Build history of the part. All positions in model axes, mm. A direction names the side the tool comes from. Give positions to 0.01 mm unless a question says otherwise; leave off trailing zeros. Write each loop counter-clockwise with the first axis right and the second up, starting at its lowest first coordinate (ties: lowest second). Pieces come first, ordered by that corner, then holes. Notation, with made-up numbers: M 86.5,65.5 L 120.5,65.5 A18 ccw 120.5,71.5 Z; hole C 26,-31.5 d8. An arc over 180 degrees is marked long. One line per item, written item: value. Start each with the question number.
Autodesk Inventor part; units mm, degrees
ref_plane "YZ Plane" through (0, 0, 0) normal (1, 0, 0) x (0, 1, 0)
ref_plane "XZ Plane" through (0, 0, 0) normal (0, 1, 0) x (-1, 0, 0)
ref_plane "XY Plane" through (0, 0, 0) normal (0, 0, 1) x (1, 0, 0)
sketch "Sketch1" plane through (0, 0, 0) normal (0, 0, 1) x (1, 0, 0)
  line L0 (-17.5, -18) -> (17.5, -18)
  line L1 (17.5, -18) -> (17.5, 18)
  line L2 (17.5, 18) -> (-17.5, 18)
  line L3 (-17.5, 18) -> (-17.5, -18)
  line L4 (-17.5, -18) -> (17.5, 18) construction
  line L5 (17.5, -18) -> (-17.5, 18) construction
  line L6 (17.5, 18) -> (2.5, 18)
  line L7 (2.5, 18) -> (2.5, 13)
  line L8 (2.5, 13) -> (17.5, 13)
  line L9 (17.5, 13) -> (17.5, 18)
  line L10 (17.5, -18) -> (2.5, -18)
  line L11 (2.5, -18) -> (2.5, -13)
  line L12 (2.5, -13) -> (17.5, -13)
  line L13 (17.5, -13) -> (17.5, -18)
  line L14 (-9, 0) -> (9, 0) construction
  line L15 (-9, -5) -> (9, -5)
  line L16 (9, 5) -> (-9, 5)
  arc A0 (-9, 5) -> (-9, -5) centre (-9, 0) ccw
  arc A1 (9, -5) -> (9, 5) centre (9, 0) ccw
  point P0 (0, 0)
  point P1 (2.5, -18)
  point P2 (17.5, 13)
  point P3 (0, 0)
  point P4 (-17.5, 0)
  dimension "d0" = 36
  dimension "d1" = 35
  dimension "d2" = 5
  dimension "d3" = 5
  dimension "d4" = 20
  dimension "d7" = 10
  dimension "d8" = 18
extrude "Extrusion1" add sketch "Sketch1" along normal blind 5 contours L3 L2 L7 L8 L1 L12 L11 L0
equation "\"d3\" = d2"
properties part number "r-support"
1) Mould opens along X. For faces 1 (the face through (17.5, 0, 2)), 2 (the face through (0, 8, 0)), 3 (the face through (14, 0, 2)) say: released by +X, released by -X, zero draft, split by the parting line, or undercut.
2) Band-saw the part on C-C (y = 0). List the corners of the cut face in (x, z).
3) Band-saw the part on A-A (x = 0.5). List the corners of the cut face in (y, z), then the cut area to 3 significant figures.
4) Drop flat-ended pins along their axis: P1, Ø1.5, axis at x = 11, z = 1.5, coming from the -Y side; P2, Ø1.5, axis at x = 9, z = 3, coming from the +Y side; P3, Ø2.5, axis at y = 15, z = 3, coming from the +X side. Give the stop position or say it passes through.
5) Probe line 1 along X through (y, z) = (3, 3.65); line 2 along Y through (x, z) = (-5, 1.15); line 3 along Y through (x, z) = (4, 4.65). List the from-to ranges inside material, lowest first. Write a range as from..to.
6) Tool access for faces 4 (the face through (10, -13, 2)), 5 (the face through (0, 5, 2)), 6 (the face through (10, 13, 2)): list every direction of +Z, -Z, +X, -X, +Y, -Y with a clear straight run to the whole face (end or side of a thin tool).
7) Band-saw the part on B-B (z = 1.2). List the corners of the cut face in (x, y).
Model answer:
1. face 1: released by +X
1. face 2: zero draft
1. face 3: undercut
2. outline: M -17.5,0 L -14,0 L -14,5 L -17.5,5 Z; M 14,0 L 17.5,0 L 17.5,5 L 14,5 Z
3. outline: M -18,0 L -5,0 L -5,5 L -18,5 Z; M 5,0 L 18,0 L 18,5 L 5,5 Z
3. area: 130 mm²
4. P1: stops at y = -13
4. P2: stops at y = 13
4. P3: stops at x = 2.5
5. line 1: x = -17.5..-13, 13..17.5
5. line 2: y = -18..-5, 5..18
5. line 3: y = -13..-5, 5..13
6. face 4: +Z, -Z, +X, -Y
6. face 5: +Z, -Z
6. face 6: +Z, -Z, +X, +Y
7. outline: M -17.5,-18 L 2.5,-18 L 2.5,-13 L 17.5,-13 L 17.5,13 L 2.5,13 L 2.5,18 L -17.5,18 Z; hole M -9,-5 L 9,-5 A5 ccw 9,5 L -9,5 A5 ccw Z
